Here's the drawing with two shaded views (mm, measured from the low corner). I have some questions. Give positions to 0.01 mm unless a question says otherwise; leave off trailing zeros. Loops run counter-clockwise (first coordinate to the right, second up) from the corner with the lowest first, then second, coordinate; pieces in that order, holes last. Notation, with made-up numbers: (-1.75, 16) - (39.25, 16) arc R22 ccw to (39.25, 41) - close; hole circle Ø8 at (-30.5, 14). An arc over 180 degrees is marked (long way). Use one line per item in the form item = value.
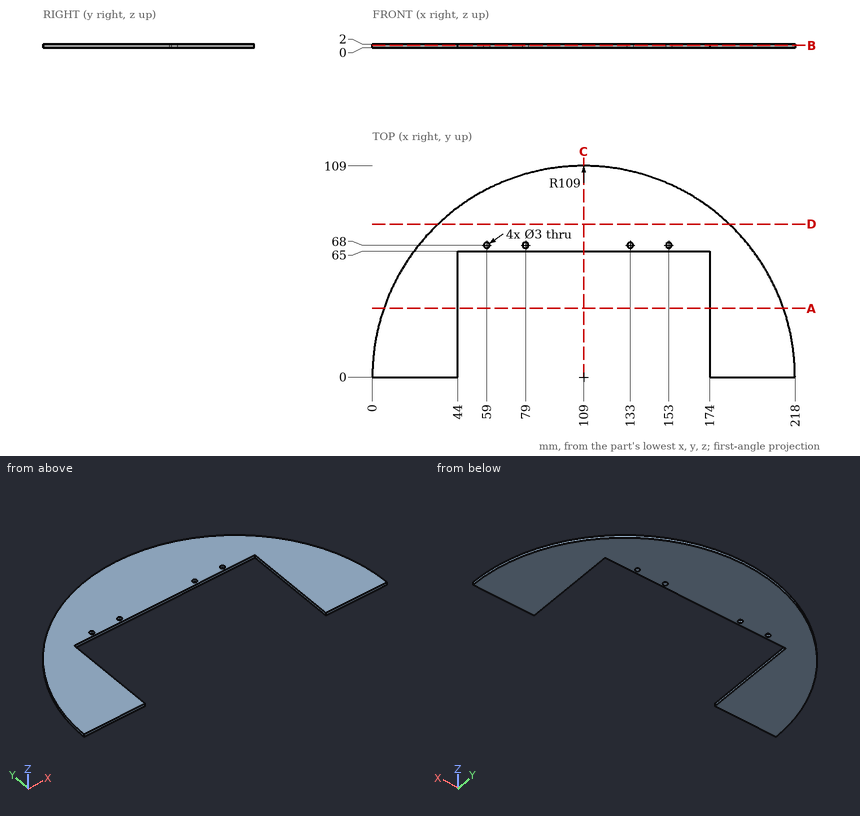
(1) If we section it at B-B (z = 1.35): List the corners of the cut face in (x, y) for me, plus the area to 3 significant figures.
Geometry says:
outline = (0, 0) - (44, 0) - (44, 65) - (174, 65) - (174, 0) - (218, 0) arc R109 ccw to start; hole circle Ø3 at (59, 68); hole circle Ø3 at (79, 68); hole circle Ø3 at (133, 68); hole circle Ø3 at (153, 68)
area = 10,200 mm²
(2) For P1, Ø1, axis at y = 48.5, z = 1.5, coming from the -X side; P2, Ø1, axis at x = 86.5, z = 1, coming from the -Y side, each with a flat end and sliding along its axis, tell me the tip position at first contact or that it passes through.
Geometry says:
P1 = 11.14
P2 = 65
(3) If we section it at D-D (y = 79): List the corners of the cut face in (x, z) for me.
Geometry says:
outline = (33.9, 0) - (184.1, 0) - (184.1, 2) - (33.9, 2) - close
(4) If we section it at A-A (y = 35.5): List the corners of the cut face in (x, z) for me.
Geometry says:
outline = (5.94, 0) - (44, 0) - (44, 2) - (5.94, 2) - close; (174, 0) - (212.06, 0) - (212.06, 2) - (174, 2) - close
(5) If I drill on probe 1 along X at (y, z) = (68, 1.3); probe 2 along Y at (x, z) = (58.5, 0.3); probe 3 along X at (y, z) = (14.5, 0.4), over which ranges is the centre line in solid material (lowest first)?
Geometry says:
probe_1 = 23.81 to 57.5, 60.5 to 77.5, 80.5 to 131.5, 134.5 to 151.5, 154.5 to 194.19
probe_2 = 65 to 66.59, 69.41 to 96.6
probe_3 = 0.97 to 44, 174 to 217.03
(6) If we section it at C-C (x = 109): List the corners of the cut face in (y, z) for me.
Geometry says:
outline = (65, 0) - (109, 0) - (109, 2) - (65, 2) - close
